Verification items for the finished model (mm, model axes). Round coordinates to 2 decimals unless told otherwise and drop trailing zeros. Write each loop counter-clockwise with the first axis right and the second up, starting at its lowest first coordinate (ties: lowest second). Pieces come first, ordered by that corner, then holes.
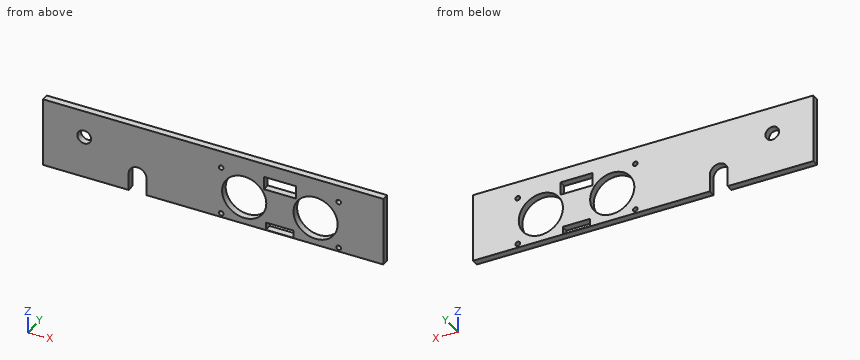
from build123d import *

# Parameters (mm, degrees)
F0_R     = 0.85
F0_R_2   = 8.05
F0_R_3   = 2.5
F1_DEPTH = 2.5


with BuildPart() as f1:
    # F0 (on Front) → F1 (new body)
    with BuildSketch(Plane.XZ):
        with BuildLine():
            Line((0, 46.5), (0, 21))
            Line((0, 21), (31.21, 21))
            Line((31.21, 21), (31.21, 27.5))
            ThreePointArc((31.21, 27.5), (34.46, 30.75), (37.71, 27.5))
            Line((37.71, 27.5), (37.71, 21))
            Line((37.71, 21), (124, 21))
            Line((124, 21), (124, 46.5))
            Line((124, 46.5), (0, 46.5))
        make_face()
        with Locations((64.88, 22.46)):
            Circle(F0_R, mode=Mode.SUBTRACT)
        Polygon((81.29, 21.16), (81.29, 23.96), (86.29, 23.96), (91.29, 23.96), (91.29, 21.16), (86.29, 21.16), align=None, mode=Mode.SUBTRACT)
        with Locations((107.7, 22.46)):
            Circle(F0_R, mode=Mode.SUBTRACT)
        with Locations((73.29, 31.33)):
            Circle(F0_R_2, mode=Mode.SUBTRACT)
        with Locations((99.29, 31.33)):
            Circle(F0_R_2, mode=Mode.SUBTRACT)
        with Locations((15, 36.5)):
            Circle(F0_R_3, mode=Mode.SUBTRACT)
        Polygon((80.49, 36.7), (80.49, 41.5), (86.29, 41.5), (92.09, 41.5), (92.09, 36.7), (86.29, 36.7), align=None, mode=Mode.SUBTRACT)
        with Locations((64.88, 40.2)):
            Circle(F0_R, mode=Mode.SUBTRACT)
        with Locations((107.7, 40.2)):
            Circle(F0_R, mode=Mode.SUBTRACT)
    extrude(amount=F1_DEPTH)


solid = f1.part
Q1. Sectioned sample at B-B (y = -0.55). Give the number of separate pieces and of enclosed holes in the cut face, plus the area to 3 significant figures.
Recorded:
separate pieces: 1
enclosed holes: 9
area: 2,580 mm2
Q2. Sectioned sample at D-D (x = 15). Enter the section's corners in (y, z).
Recorded:
outline: (-2.5, 21) - (0, 21) - (0, 34) - (-2.5, 34) - close; (-2.5, 39) - (0, 39) - (0, 46.5) - (-2.5, 46.5) - close
Q3. Sectioned sample at A-A (x = 73.29). Enter the section's corners in (y, z).
Recorded:
outline: (-2.5, 21) - (0, 21) - (0, 23.28) - (-2.5, 23.28) - close; (-2.5, 39.38) - (0, 39.38) - (0, 46.5) - (-2.5, 46.5) - close
Q4. Sectioned sample at C-C (z = 25.75). Enter the section's corners in (x, y).
Recorded:
outline: (0, -2.5) - (31.21, -2.5) - (31.21, 0) - (0, 0) - close; (37.71, -2.5) - (67.49, -2.5) - (67.49, 0) - (37.71, 0) - close; (79.09, -2.5) - (93.49, -2.5) - (93.49, 0) - (79.09, 0) - close; (105.09, -2.5) - (124, -2.5) - (124, 0) - (105.09, 0) - close
Q5. Material ranges on line 1 along Z through (x, y) = (107.7, -0.75); line 2 along Z through (x, y) = (91, -0.6); line 3 along Z through (x, y) = (73.29, -0.65), recorded low to high.
Recorded:
line 1: z = 21 to 21.61, 23.31 to 39.35, 41.05 to 46.5
line 2: z = 21 to 21.16, 23.96 to 36.7, 41.5 to 46.5
line 3: z = 21 to 23.28, 39.38 to 46.5
